Source: CAD feature listing. Evaluate the final solid. Frame: model axes, mm. A direction names the side the tool comes from. Give positions to 0.01 mm unless a question says otherwise; leave off trailing zeros. Write each loop counter-clockwise with the first axis right and the second up, starting at its lowest first coordinate (ties: lowest second). Pieces come first, ordered by that corner, then holes. Notation, with made-up numbers: (80, 27) -> (86, 27) arc R25 cw to (86, 66) -> close; hole circle Ø7 at (27.25, 26.5). An arc over 180 degrees is marked (long way). Write item = value, one per line.
from build123d import *

# Parameters (mm, degrees)
F1_DEPTH = 3.175
F3_D     = 4.7625
F4_R     = 5.08


with BuildPart() as f1:
    # F0 (on Top) → F1 (new body)
    with BuildSketch(Plane.XY):
        Polygon((63.5, 0), (0, 0), (0, -127), (127, -127), (127, -63.5), (63.5, -63.5), align=None)
    extrude(amount=F1_DEPTH)

    # F3 (through all)
    with Locations(Plane.XY.offset(3.175)):
        with Locations((12.7, -12.7), (50.8, -12.7), (50.8, -50.8), (12.7, -88.9), (38.1, -114.3), (76.2, -76.2), (114.3, -76.2), (114.3, -114.3)):
            Hole(F3_D / 2)

    # F4
    f4_edges = [f1.edges().sort_by_distance(p)[0] for p in [
        (63.5, -63.5, 1.5875),
        (63.5, 0, 1.5875),
        (0, 0, 1.5875),
        (127, -63.5, 1.5875),
        (127, -127, 1.5875),
        (0, -127, 1.5875),
    ]]
    fillet(f4_edges, radius=F4_R)


solid = f1.part
(1) Section query D-D (z = 2.3). Give the number of separate pieces and of enclosed holes in the cut face, plus the area to 3 significant figures.
Values follow:
separate_pieces = 1
enclosed_holes = 8
area = 11,900 mm2
(2) Pull-direction query (X, two-part tool) for faces 3 (the face through (0, -63, 2)), 4 (the face through (13.01, -86.54, 1.57)), 5 (the face through (64.949, -61.972, 1.61)); classes: pulls with the +X half, pulls with the -X half, needs draft (parallel to the pull), parting line crosses it, or undercut.
Values follow:
face_3 = pulls with the -X half
face_4 = undercut
face_5 = pulls with the +X half
(3) First-contact query: pin 1 (1 mm diameter, centred on x = 88.5, z = 1, fed in from +Y). Flat tip, straight axial feed; report the tip coordinate or a pass-through.
Values follow:
pin_1 = -63.5
(4) Material intervals for line 1 (Y direction, x = 12.7, z = 1.15); line 2 (Y direction, x = 114.3, z = 0.85); line 3 (X direction, y = -25, z = 2.45), sorted ascending.
Values follow:
line_1 = -127 to -91.28, -86.52 to -15.08, -10.32 to 0
line_2 = -127 to -116.68, -111.92 to -78.58, -73.82 to -63.5
line_3 = 0 to 63.5
(5) Access query for faces 1 (the face through (96, -63.5, 2)), 2 (the face through (125.472, -125.551, 1.61)). Directions: +Z, -Z, +X, -X, +Y, -Y. A direction counts if a zero-diameter tool reaches every point of the face in a straight line with its end or side. Return the directions, or none.
Values follow:
face_1 = +Z, -Z, +X, +Y
face_2 = +Z, -Z, +X, -Y
(6) Section query A-A (y = -114.3). Return loops of the section in (x, z) (3 decimals), plus the area to 3 significant figures.
Values follow:
outline = (0, 0) -> (35.719, 0) -> (35.719, 3.175) -> (0, 3.175) -> close; (40.481, 0) -> (111.919, 0) -> (111.919, 3.175) -> (40.481, 3.175) -> close; (116.681, 0) -> (127, 0) -> (127, 3.175) -> (116.681, 3.175) -> close
area = 373 mm2
(7) Section query C-C (y = -50.8). Return loops of the section in (x, z) (3 decimals), plus the area to 3 significant figures.
Values follow:
outline = (0, 0) -> (48.419, 0) -> (48.419, 3.175) -> (0, 3.175) -> close; (53.181, 0) -> (63.5, 0) -> (63.5, 3.175) -> (53.181, 3.175) -> close
area = 186 mm2
(8) Section query B-B (x = 114.3). Return loops of the section in (y, z) (3 decimals).
Values follow:
outline = (-127, 0) -> (-116.681, 0) -> (-116.681, 3.175) -> (-127, 3.175) -> close; (-111.919, 0) -> (-78.581, 0) -> (-78.581, 3.175) -> (-111.919, 3.175) -> close; (-73.819, 0) -> (-63.5, 0) -> (-63.5, 3.175) -> (-73.819, 3.175) -> close
